from build123d import *

# Parameters (mm, degrees)
F1_DEPTH = 25.4


with BuildPart() as f1:
    # F0 (on Front) → F1 (new body)
    with BuildSketch(Plane.XZ):
        with BuildLine():
            add(Edge.make_bspline(
                [(-41.275, 9.525), (-19.526121, 41.756507), (15.662241, 57.34362), (52.757816, 61.879481)],
                knots=[0, 0, 0, 0, 107.612327, 107.612327, 107.612327, 107.612327], degree=3))
            Line((-41.275, 9.525), (22.225, 9.525))
            Line((22.225, 9.525), (22.225, 27.231764))
            ThreePointArc((22.225, 27.231764), (30.947399, 50.322439), (52.757816, 61.879481))
        make_face()
        Polygon((22.225, 9.525), (-41.275, 9.525), (-41.275, -9.525), (41.275, -9.525), (41.275, 9.525), align=None)
        with BuildLine():
            Line((22.225, 27.231764), (22.225, 9.525))
            Line((22.225, 9.525), (41.275, 9.525))
            Line((41.275, 9.525), (41.275, 27.231764))
            ThreePointArc((41.275, 27.231764), (45.007035, 37.457419), (54.448422, 42.8752))
            Line((54.448422, 42.8752), (60.325, 42.8752))
            Line((60.325, 42.8752), (60.325, 61.9252))
            Line((60.325, 61.9252), (53.134891, 61.9252))
            add(Edge.make_bspline(
                [(52.757816, 61.879481), (52.883486, 61.894848), (53.009178, 61.910087), (53.134891, 61.9252)],
                knots=[107.612327, 107.612327, 107.612327, 107.612327, 107.976889, 107.976889, 107.976889, 107.976889], degree=3))
            ThreePointArc((52.757816, 61.879481), (30.947399, 50.322439), (22.225, 27.231764))
        make_face()
        with BuildLine():
            ThreePointArc((53.134891, 61.9252), (52.946292, 61.902853), (52.757816, 61.879481))
            add(Edge.make_bspline(
                [(52.757816, 61.879481), (52.883486, 61.894848), (53.009178, 61.910087), (53.134891, 61.9252)],
                knots=[107.612327, 107.612327, 107.612327, 107.612327, 107.976889, 107.976889, 107.976889, 107.976889], degree=3))
        make_face()
        Polygon((60.325, 66.675), (60.325, 61.9252), (60.325, 42.8752), (85.748771, 42.8752), (85.867248, 66.675), align=None)
        Polygon((85.748771, 42.8752), (60.325, 42.8752), (60.325, 38.1), (85.725, 38.1), align=None)
        Polygon((85.867248, 66.675), (85.748771, 42.8752), (85.725, 38.1), (111.125, 38.1), (111.125, 66.675), align=None)
    extrude(amount=F1_DEPTH)


solid = f1.part
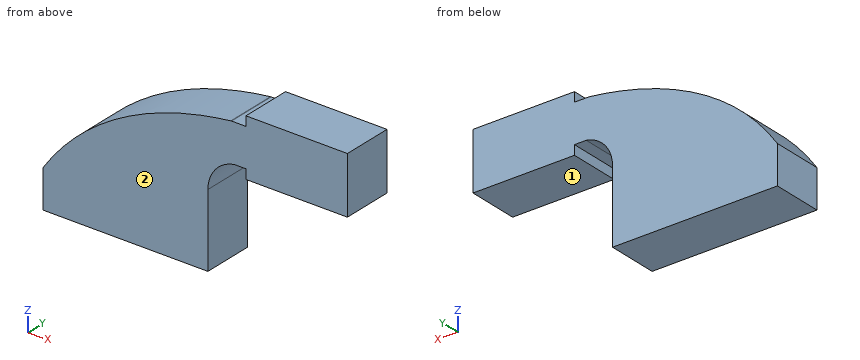
Here's how the part is built. I have some questions about the finished solid (model axes, mm). Face numbers are marked on the shaded views. A direction names the side the tool comes from. Coordinates: 2 decimals unless noted, no trailing zeros. Write each loop counter-clockwise with the first axis right and the second up, starting at its lowest first coordinate (ties: lowest second). Pieces come first, ordered by that corner, then holes.
1) If I drill on line 1 (X direction, y = -13, z = 4) (3 decimals); line 2 (Z direction, x = 70.5, y = -20) (3 decimals); line 3 (X direction, y = -20, z = 37), over which ranges is the centre line in solid material (lowest first)?
Filled in:
line 1: x = -41.275 to 41.275
line 2: z = 38.1 to 66.675
line 3: x = -14.68 to 44.64
2) Which directions (+Z, -Z, +X, -X, +Y, -Y) give clear straight access to the entire face, cutting with the end or side of a thin tool? Please do the marked faces 1 and 2.
Filled in:
face 1: -Z, +X, +Y, -Y
face 2: +Z, -Z, +X, -X, -Y
3) I'm going to push flat-ended pins straight in: pin 1 (4 mm diameter, centred on x = 35.5, y = -22.5, fed in from +Z); pin 2 (2 mm diameter, centred on y = -8.5, z = 38, fed in from -X); pin 3 (4.5 mm diameter, centred on x = 56.5, y = -9, fed in from -Z); pin 4 (6 mm diameter, centred on x = 2.5, z = 53.5, fed in from +Y). Where does each tip first touch, or does it pass through?
Filled in:
pin 1: stops at z = 59.35
pin 2: stops at x = -14.68
pin 3: stops at z = 42.84
pin 4: passes through
4) If we section it at A-A (z = 1.5): List the corners of the cut face in (x, y) for me (3 decimals).
Filled in:
outline: (-41.275, -25.4) - (41.275, -25.4) - (41.275, 0) - (-41.275, 0) - close
5) If we section it at B-B (x = 95): List the corners of the cut face in (y, z) for me (3 decimals), plus the area to 3 significant figures.
Filled in:
outline: (-25.4, 38.1) - (0, 38.1) - (0, 66.675) - (-25.4, 66.675) - close
area: 726 mm2
